The model under review builds one solid part; all positions refer to its coordinate system, in mm. Face numbers are marked on the shaded views. A direction names the side the tool comes from. Coordinates: 2 decimals unless noted, no trailing zeros. Loops run counter-clockwise (first coordinate to the right, second up) from the corner with the lowest first, then second, coordinate; pieces in that order, holes last. Notation, with made-up numbers: (10.5, 64.25) -> (36.5, 64.25) arc R17 cw to (36.5, 75.25) -> close; hole circle Ø7 at (65, 19.5). An arc over 180 degrees is marked (long way). One line per question, with ' | ' between items. Start each with the question number.
from build123d import *

# Parameters (mm, degrees)
F0_R          = 11.43
F1_DEPTH      = 76.2
F3_START      = 15.24
F2_R          = 19.05
F3_DEPTH      = 5.08
F4_W          = 215.9
F4_H          = 22.86
F4_R          = 5.08
F5_DEPTH      = 7.5
F2_W          = 63.5
F2_H          = 63.5
F2_R_2        = 22.225
F6_DEPTH      = 0.508
F6_DEPTH_BACK = 7.62
F8_START      = 82.55
F7_W          = 40
F7_H          = 40
F7_R          = 15
F8_DEPTH      = 25.4
F9_START      = 107.95
F9_DEPTH      = 50.8
F10_START     = -82.55
F10_DEPTH     = 25.4
F11_START     = -107.95
F11_DEPTH     = 50.8


with BuildPart() as f1:
    # F0 (on Top) → F1 (new body)
    with BuildSketch(Plane.XY):
        Circle(F0_R)
    extrude(amount=F1_DEPTH)

    # F2 (on Top) → F3 (join)
    with BuildSketch(Plane.XY.offset(F3_START)):
        Circle(F2_R)
    extrude(amount=F3_DEPTH)

    # F4 (on Top) → F5 (join)
    with BuildSketch(Plane.XY):
        Rectangle(F4_W, F4_H)
        with Locations((-97.79, 0)):
            Circle(F4_R, mode=Mode.SUBTRACT)
        with Locations((97.79, 0)):
            Circle(F4_R, mode=Mode.SUBTRACT)
    extrude(amount=-F5_DEPTH)

    # F2 (on Top) → F6 (join, two sides)
    with BuildSketch(Plane.XY) as f6_sk:
        Rectangle(F2_W, F2_H)
        Circle(F2_R_2, mode=Mode.SUBTRACT)
        Circle(F2_R_2)
        Circle(F2_R, mode=Mode.SUBTRACT)
        Circle(F2_R)
    extrude(amount=F6_DEPTH)
    extrude(f6_sk.sketch, amount=-F6_DEPTH_BACK)

    # F7 (on Right) → F8 (join)
    with BuildSketch(Plane.YZ.offset(F8_START)):
        with Locations((0, -20)):
            Rectangle(F7_W, F7_H)
        with Locations((0, -20)):
            Circle(F7_R, mode=Mode.SUBTRACT)
        with Locations((0, -20)):
            Circle(F7_R)
    extrude(amount=F8_DEPTH)

    # F7 (on Right) → F9 (join)
    with BuildSketch(Plane.YZ.offset(F9_START)):
        with Locations((0, -20)):
            Circle(F7_R)
    extrude(amount=F9_DEPTH)

    # F7 (on Right) → F10 (join)
    with BuildSketch(Plane.YZ.offset(F10_START)):
        with Locations((0, -20)):
            Rectangle(F7_W, F7_H)
        with Locations((0, -20)):
            Circle(F7_R, mode=Mode.SUBTRACT)
        with Locations((0, -20)):
            Circle(F7_R)
    extrude(amount=-F10_DEPTH)

    # F7 (on Right) → F11 (join)
    with BuildSketch(Plane.YZ.offset(F11_START)):
        with Locations((0, -20)):
            Circle(F7_R)
    extrude(amount=-F11_DEPTH)


solid = f1.part
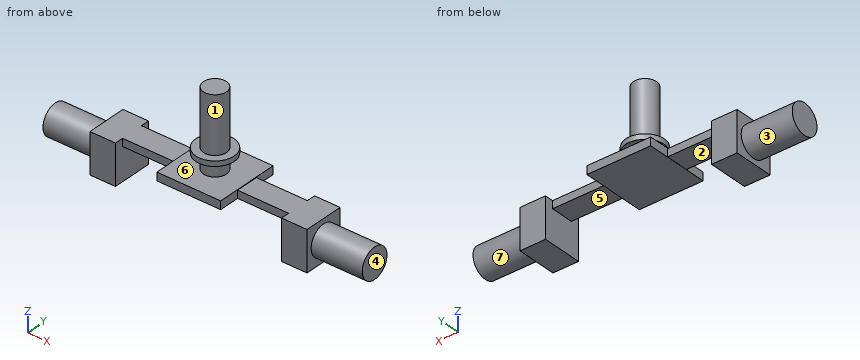
1) Consider section D-D, the plane z = 6. Write out the cut boundary in (x, y), plus the area to 3 significant figures.
2) Consider section A-A, the plane z = -20. Write out the cut boundary in (x, y), plus the area to 3 significant figures.
3) Wall thickness on L1, parallel to X at y = 8, z = -20; L2, parallel to X at y = -10, z = -33.5; L3, parallel to Z at x = 28, y = 19: over which ranges is each line inside the solid? List them lowest first.
4) Consider section C-C, the plane y = -24. Write out the cut boundary in (x, z), plus the area to 3 significant figures.
5) Insertion check: pin 1 Ø2 at (x, z) = (41.5, 0.5) entering from -Y; pin 2 Ø8 at (x, y) = (5, 8.5) entering from -Z; pin 3 Ø6 at (x, z) = (-15.5, 11.5) entering from -Y; pin 4 Ø11.5 at (x, y) = (-69.5, 2) entering from -Z. Each pin has a flat end and moves straight along its axis. Give the tip position at first contact, or say it passes through.
6) Consider section B-B, the plane x = 0. Write out the cut boundary in (y, z).
7) Mouldability with a two-part tool opening along X and no side actions: class the marked faces 1, 2, 3 and 4 as +X half, -X half, draft (parallel to the pull), parting line (faces both ways), or undercut.
8) Machinability: for the marked faces 5, 6 and 7, which of the approach directions +Z, -Z, +X, -X, +Y, -Y give a long, thin tool a straight path to every point of the face, cutting with its end or side? Answer none if there is none.
Filled sheet:
1) outline: circle Ø22.86 at (0, 0) | area: 410 mm^2
2) outline: (-158.75, -15) -> (-107.95, -15) -> (-107.95, -20) -> (-82.55, -20) -> (-82.55, 20) -> (-107.95, 20) -> (-107.95, 15) -> (-158.75, 15) -> close; (82.55, -20) -> (107.95, -20) -> (107.95, -15) -> (158.75, -15) -> (158.75, 15) -> (107.95, 15) -> (107.95, 20) -> (82.55, 20) -> close | area: 5,080 mm^2
3) L1: -158.75 to -82.55, 82.55 to 158.75 | L2: -107.95 to -82.55, 82.55 to 107.95 | L3: -7.62 to 0.51
4) outline: (-31.75, -7.62) -> (31.75, -7.62) -> (31.75, 0.51) -> (-31.75, 0.51) -> close | area: 516 mm^2
5) pin 1: y = -11.43 | pin 2: z = -7.62 | pin 3: through | pin 4: z = -7.5
6) outline: (-31.75, -7.62) -> (31.75, -7.62) -> (31.75, 0.51) -> (11.43, 0.51) -> (11.43, 15.24) -> (19.05, 15.24) -> (19.05, 20.32) -> (11.43, 20.32) -> (11.43, 76.2) -> (-11.43, 76.2) -> (-11.43, 20.32) -> (-19.05, 20.32) -> (-19.05, 15.24) -> (-11.43, 15.24) -> (-11.43, 0.51) -> (-31.75, 0.51) -> close
7) face 1: parting line | face 2: undercut | face 3: draft | face 4: +X half
8) face 5: -Z, +Y, -Y | face 6: none | face 7: +X
